Verification items for the finished model (mm, model axes). A direction names the side the tool comes from. Give positions to 0.01 mm unless a question says otherwise; leave off trailing zeros. Order: outer loops, then holes, each group sorted by start corner. A loop starts at its lowest first (then second) coordinate and runs counter-clockwise, first axis right, second up.
(1) Access from +Z, -Z, +X, -X, +Y, -Y to the whole of each face (thin tool, end or side, straight path). Record for faces 4 (the face through (89.08, -3.13, 18.87)), 5 (the face through (52.516, -3.131, -1.808)).
(2) Sectioned sample at C-C on z = -15.5. Record the cut outline in (x, y), plus the area to 3 significant figures.
(3) Gauge pin test, flat end, axial feed: pin 1 (6.5 mm diameter, centred on x = -2.66, z = 12.7, fed in from -Y). Record the tip position at first contact, or that the pin passes through.
(4) Sectioned sample at A-A on x = 82.55. Record the cut outline in (y, z).
(5) Scan lines: L1, parallel to X at y = -1, z = 0.5; L2, parallel to Z at x = -54.5, y = -4; L3, parallel to X at y = -1.25, z = -3.5. Record each from-to range of solid material in increasing order.
(6) Mould release check, pull along Z, two halves, no side actions. Record for faces 1 (the face through (-81.09, -3.13, 3.43)), 2 (the face through (-1, -3, -31.75)), 3 (the face through (-11, -3, 31.75)): pulls with the +Z half, pulls with the -Z half, needs draft (parallel to the pull), parting line crosses it, or undercut.
(7) Sectioned sample at B-B on y = -4.75. Count the separate pieces of the cut face and the enclosed holes in it, plus the area to 3 significant figures.
```python
from build123d import *

# Parameters (mm, degrees)
F1_DEPTH = 6.35


with BuildPart() as f1:
    # F0 (on Front) → F1 (new body)
    with BuildSketch(Plane.XZ):
        Polygon((-101.6, -31.75), (101.6, -31.75), (101.6, 6.35), (76.2, 31.75), (-101.6, 31.75), align=None)
        with BuildLine():
            ThreePointArc((77.225286, -11.11276), (83.352019, -7.201939), (88.10625, -12.7))
            ThreePointArc((88.10625, -12.7), (81.747981, -18.198061), (77.225286, -11.11276))
        make_face(mode=Mode.SUBTRACT)
        with BuildLine():
            ThreePointArc((-82.541162, 0.290002), (-81.050955, 3.468612), (-77.7875, 4.7625))
            Line((-77.7875, 4.7625), (-8.989503, 4.7625))
            ThreePointArc((-8.989503, 4.7625), (-5.621907, 3.367596), (-4.227003, 0))
            ThreePointArc((-4.227003, 0), (-5.621907, -3.367596), (-8.989503, -4.7625))
            Line((-8.989503, -4.7625), (-77.7875, -4.7625))
            ThreePointArc((-77.7875, -4.7625), (-81.155096, -3.367596), (-82.55, 0))
            ThreePointArc((-82.55, 0), (-82.54779, 0.145068), (-82.541162, 0.290002))
        make_face(mode=Mode.SUBTRACT)
        with BuildLine():
            ThreePointArc((2.89687, 12.7), (2.838681, 11.897981), (2.665334, 11.11276))
            ThreePointArc((2.665334, 11.11276), (-8.157441, 13.502019), (2.89687, 12.7))
        make_face(mode=Mode.SUBTRACT)
        with BuildLine():
            ThreePointArc((52.64531, 0), (52.512307, -1.833187), (52.116086, -3.627977))
            ThreePointArc((52.116086, -3.627977), (36.317333, -12.170776), (27.774534, 3.627977))
            ThreePointArc((27.774534, 3.627977), (41.778497, 12.566997), (52.64531, 0))
        make_face(mode=Mode.SUBTRACT)
    extrude(amount=F1_DEPTH)


solid = f1.part
```
Ans:
1. face 4: +Z, +X, +Y, -Y
1. face 5: +Y, -Y
2. outline: (-101.6, -6.35) - (77.75, -6.35) - (77.75, 0) - (-101.6, 0) - close; (87.35, -6.35) - (101.6, -6.35) - (101.6, 0) - (87.35, 0) - close
2. area: 1,230 mm2
3. pin 1: passes through
4. outline: (-6.35, -31.75) - (0, -31.75) - (0, -18.26) - (-6.35, -18.26) - close; (-6.35, -7.14) - (0, -7.14) - (0, 25.4) - (-6.35, 25.4) - close
5. L1: x = -101.6 to -82.52, -4.25 to 27.26, 52.64 to 101.6
5. L2: z = -31.75 to -4.76, 4.76 to 31.75
5. L3: x = -101.6 to -81.02, -5.76 to 27.74, 52.15 to 101.6
6. face 1: undercut
6. face 2: pulls with the -Z half
6. face 3: pulls with the +Z half
7. separate pieces: 1
7. enclosed holes: 4
7. area: 11,200 mm2
